Part model, mm, in its own coordinate system. A direction names the side the tool comes from. Round coordinates to 2 decimals unless told otherwise and drop trailing zeros. Loops run counter-clockwise (first coordinate to the right, second up) from the corner with the lowest first, then second, coordinate; pieces in that order, holes last. Notation, with made-up numbers: (12.5, -40) - (17.5, -40) arc R14 cw to (17.5, -34) - close; hole circle Ø9 at (3, -36.75). An arc over 180 degrees is marked (long way). Write each question's results on one line, items separated by ' | '. Start each with the question number.
(1) Cut at B-B, the plane y = 60.5. List the corners of the cut face in (x, z).
(2) Mould opens along Z. For faces 1 (the face through (-23.28, 1.48, 12.12)), 2 (the face through (10.51, 1.48, 9.17)), 3 (the face through (5, 56, 0)), 4 (the face through (-0.27, 1.48, -28.78)) say: released by +Z, released by -Z, zero draft, split by the parting line, or undercut.
(3) Cut at D-D, the plane y = 9. List the corners of the cut face in (x, z), then the cut area to 3 significant figures.
(4) Flat gauge pins, fed straight in: P1, Ø8, axis at x = -0.5, y = 57, coming from the -Z side; P2, Ø2.5, axis at x = 1, z = -15.5, coming from the +Y side; P3, Ø10.5, axis at x = -20.5, z = 7, coming from the +Y side; P4, Ø11, axis at x = 2, z = -9.5, coming from the -Y side. Where does each tip first touch, or does it go through?
(5) Cut at A-A, the plane z = -30. List the corners of the cut face in (x, y).
(6) Tool access for faces 5 (the face through (22.135, 1.479, 14.103)), 6 (the face through (-5, 54, 0)), 7 (the face through (2.69, 1.48, -13.68)): list every direction of +Z, -Z, +X, -X, +Y, -Y with a clear straight run to the whole face (end or side of a thin tool).
(7) Cut at C-C, the plane z = 10. List the corners of the cut face in (x, y), then the cut area to 3 significant figures.
(8) Drill centre lines: L1, parallel to Z at x = 3.2, y = 64; L2, parallel to Y at x = 3, z = -14; L3, parallel to Z at x = 0, y = 0.6. Where is each one in solid material? Low to high.
from build123d import *

# Parameters (mm, degrees)
SKETCH1_W                = 5
SKETCH1_H                = 50
SKETCH2_R                = 1.25
BOSS_EXTRUDE1_DEPTH      = 3
CIRPATTERN1_COUNT        = 3
BOSS_EXTRUDE2_DEPTH      = 5
BOSS_EXTRUDE2_DEPTH_BACK = 5
SKETCH3_3_W              = 6
SKETCH3_3_H              = 12
SKETCH3_3_R              = 1.5
BOSS_EXTRUDE3_DEPTH      = 5
SKETCH4_W                = 2.5
SKETCH4_H                = 12
CUT_EXTRUDE1_DEPTH       = 52


with BuildPart() as part:
    # Sketch1 → Revolve1 (revolve)
    with BuildSketch(Plane.XY):
        with Locations((2.5, 25)):
            Rectangle(SKETCH1_W, SKETCH1_H)
    revolve(axis=Axis((0, 0, 0), (0, 1, 0)))

    # Sketch2 → Boss-Extrude1 (add)
    with BuildSketch(Plane(origin=(0, 0, 0), x_dir=(1, 0, 0), z_dir=(0, 1, 0))):
        with BuildLine():
            ThreePointArc((1, 25.183337145), (1.152197325, 26.235023126), (1.855037693, 27.032031813))
            ThreePointArc((1.855037693, 27.032031813), (0, 33.5), (-1.855037693, 27.032031813))
            ThreePointArc((-1.855037693, 27.032031813), (-1.152197325, 26.235023126), (-1, 25.183337145))
            Line((-1, 25.183337145), (-4.330127019, 2.5))
            Line((-4.330127019, 2.5), (4.330127019, 2.5))
            Line((4.330127019, 2.5), (1, 25.183337145))
        make_face()
        with Locations((0, 30)):
            Circle(SKETCH2_R, mode=Mode.SUBTRACT)
    boss_extrude1 = extrude(amount=BOSS_EXTRUDE1_DEPTH)

    # CirPattern1: Boss-Extrude1 ×3 about axis
    cirpattern1_axis = Axis((0, 0, 0), (0, 1, 0))
    for i in range(1, CIRPATTERN1_COUNT):
        add(boss_extrude1.rotate(cirpattern1_axis, i * 360 / CIRPATTERN1_COUNT))

    # Sketch3 → Boss-Extrude2 (add, two sides)
    with BuildSketch(Plane(origin=(0, 0, 0), x_dir=(0, 0, -1), z_dir=(1, 0, 0))) as boss_extrude2_sk:
        Polygon((-17.5, 50), (17.5, 50), (17.5, 58), (11.5, 58), (-11.5, 58), (-17.5, 58), align=None)
    extrude(amount=BOSS_EXTRUDE2_DEPTH)
    extrude(boss_extrude2_sk.sketch, amount=-BOSS_EXTRUDE2_DEPTH_BACK)

    # Sketch3_3 → Boss-Extrude3 (add)
    with BuildSketch(Plane(origin=(0, 0, 0), x_dir=(0, 0, -1), z_dir=(1, 0, 0))):
        with Locations((-14.5, 64)):
            Rectangle(SKETCH3_3_W, SKETCH3_3_H)
        with Locations((-14, 64)):
            Circle(SKETCH3_3_R, mode=Mode.SUBTRACT)
        with Locations((14.5, 64)):
            Rectangle(SKETCH3_3_W, SKETCH3_3_H)
        with Locations((14, 64)):
            Circle(SKETCH3_3_R, mode=Mode.SUBTRACT)
    extrude(amount=BOSS_EXTRUDE3_DEPTH)

    # Sketch4 → Cut-Extrude1 (cut, through all)
    with BuildSketch(Plane.XY.offset(17.5)):
        with Locations((1.25, 64)):
            Rectangle(SKETCH4_W, SKETCH4_H)
    extrude(amount=-CUT_EXTRUDE1_DEPTH, mode=Mode.SUBTRACT)


solid = part.part
A:
1) outline: (2.5, -17.5) - (5, -17.5) - (5, -11.5) - (2.5, -11.5) - close; (2.5, 11.5) - (5, 11.5) - (5, 17.5) - (2.5, 17.5) - close
2) face 1: released by -Z | face 2: released by +Z | face 3: zero draft | face 4: undercut
3) outline: circle Ø10 at (0, 0) | area: 78.5 mm2
4) P1: z = -17.5 | P2: y = 58 | P3: y = 3 | P4: y = 0
5) outline: (-3.5, 0) - (-1.25, 0) - (-1.25, 3) - (-3.5, 3) - close; (1.25, 0) - (3.5, 0) - (3.5, 3) - (1.25, 3) - close
6) face 5: +Z, +Y, -Y | face 6: +Z, -Z, -X, +Y | face 7: +X, -Y
7) outline: (-20.13, 0) - (-12.6, 0) - (-12.6, 3) - (-20.13, 3) - close; (-5, 50) - (5, 50) - (5, 58) - (-5, 58) - close; (12.6, 0) - (20.13, 0) - (20.13, 3) - (12.6, 3) - close | area: 125 mm2
8) L1: -17.5 to -15.5, -12.5 to -11.5, 11.5 to 12.5, 15.5 to 17.5 | L2: 50 to 62.5, 65.5 to 70 | L3: -33.5 to -31.25, -28.75 to 5
